Read the model definition and answer for the solid it produces. Units are mm, in the model's axes. A direction names the side the tool comes from. Coordinates: 2 decimals unless noted, no trailing zeros. Write each loop counter-clockwise with the first axis right and the second up, starting at its lowest first coordinate (ties: lowest second). Pieces come first, ordered by that corner, then holes.
Item 1: Section A-A (x = 2.5) is taken. Give the vertices of the cut face in (y, z), then the cut area to 3 significant figures.
Item 2: A tool of negligible diameter and unlimited length cuts with its end or side. For faces 4 (the face through (12, 1, -28)), 5 (the face through (37, 3, -17)), from which of +Z, -Z, +X, -X, +Y, -Y can it reach the whole face along a straight path? Write none if from no direction.
Item 3: This flat-tipped pin is pushed along its axis until it touches: P1, Ø3, axis at x = 71.5, z = -30.5, coming from the -Y side. Where does it stop, or does it pass through?
Item 4: Determine the mould class of faces 1 (the face through (74, 1, -16)), 2 (the face through (36, 0, -17)), 3 (the face through (72.978, 1.014, -30.966)) for opening direction X: released by +X, released by -X, zero draft, split by the parting line, or undercut.
Item 5: Section C-C (x = 61) is taken. Give the vertices of the cut face in (y, z), then the cut area to 3 significant figures.
Item 6: Straight lines are drawn through the part: probe 1 along Z at (x, y) = (71.5, 0.85); probe 2 along X at (y, z) = (1.4, -2.5); probe 3 along X at (y, z) = (0.85, -26). For each, find the intervals that lie inside material, in ascending order.
Item 7: Section B-B (z = -8) is taken. Give the vertices of the cut face in (x, y), then the cut area to 3 significant figures.
from build123d import *

# Parameters (mm, degrees)
SKETCH1_W           = 74
SKETCH1_H           = 33
BOSS_EXTRUDE1_DEPTH = 2
SKETCH2_W           = 62
SKETCH2_H           = 28
BOSS_EXTRUDE2_DEPTH = 1
SKETCH3_R           = 1.55
CUT_EXTRUDE2_DEPTH  = 5
FILLET1_R           = 0.5
FILLET2_R           = 0.5
SKETCH4_W           = 15
SKETCH4_H           = 15
CUT_EXTRUDE3_DEPTH  = 10
FILLET3_R           = 0.5


with BuildPart() as part:
    # Sketch1 → Boss-Extrude1 (new body)
    with BuildSketch(Plane(origin=(0, 0, 0), x_dir=(1, 0, 0), z_dir=(0, 1, 0))):
        with Locations((37, 16.5)):
            Rectangle(SKETCH1_W, SKETCH1_H)
    extrude(amount=BOSS_EXTRUDE1_DEPTH)

    # Sketch2 → Boss-Extrude2 (add)
    with BuildSketch(Plane(origin=(0, 2, 0), x_dir=(1, 0, 0), z_dir=(0, 1, 0))):
        with Locations((37, 16.5)):
            Rectangle(SKETCH2_W, SKETCH2_H)
    extrude(amount=BOSS_EXTRUDE2_DEPTH)

    # Sketch3 → Cut-Extrude2 (cut)
    with BuildSketch(Plane(origin=(0, 2, 0), x_dir=(1, 0, 0), z_dir=(0, 1, 0))):
        with Locations((2.5, 30.5)):
            Circle(SKETCH3_R)
        with Locations((71.5, 2.5)):
            Circle(SKETCH3_R)
        with Locations((2.5, 2.5)):
            Circle(SKETCH3_R)
        with Locations((71.5, 30.5)):
            Circle(SKETCH3_R)
    extrude(amount=-CUT_EXTRUDE2_DEPTH, mode=Mode.SUBTRACT)

    # Fillet1
    fillet1_edges = [part.edges().sort_by_distance(p)[0] for p in [
        (6, 3, -16.5),
        (37, 3, -2.5),
        (68, 3, -16.5),
        (37, 3, -30.5),
    ]]
    fillet(fillet1_edges, radius=FILLET1_R)

    # Fillet2
    fillet2_edges = [part.edges().sort_by_distance(p)[0] for p in [
        (37, 0, -33),
        (74, 0, -16.5),
        (37, 0, 0),
        (0, 0, -16.5),
        (0, 1, -33),
        (74, 1, -33),
        (74, 1, 0),
        (0, 1, 0),
    ]]
    fillet(fillet2_edges, radius=FILLET2_R)

    # Sketch4 → Cut-Extrude3 (cut)
    with BuildSketch(Plane.XZ):
        with Locations((12.5, -20.5)):
            Rectangle(SKETCH4_W, SKETCH4_H)
    extrude(amount=-CUT_EXTRUDE3_DEPTH, mode=Mode.SUBTRACT)

    # Fillet3
    fillet3_edges = [part.edges().sort_by_distance(p)[0] for p in [
        (13.25, 3, -13),
        (20, 1.5, -13),
        (13.25, 3, -28),
        (5, 0, -20.5),
        (12.5, 0, -28),
        (20, 0, -20.5),
        (12.5, 0, -13),
        (6.146446609, 2.853553391, -28),
        (6.146446609, 2.853553391, -13),
        (20, 3, -20.5),
        (5, 2, -20.5),
        (5, 1, -28),
        (6, 2.25, -13),
        (5.5, 2, -13),
        (5, 1, -13),
        (5.5, 2, -28),
        (6, 2.25, -28),
        (20, 1.5, -28),
    ]]
    fillet(fillet3_edges, radius=FILLET3_R)


solid = part.part
Established:
1. outline: (0, -32.5) arc R0.5 ccw to (0.5, -33) - (2, -33) - (2, -32.05) - (0, -32.05) - close; (0, -28.95) - (2, -28.95) - (2, -4.05) - (0, -4.05) - close; (0, -0.95) - (2, -0.95) - (2, 0) - (0.5, 0) arc R0.5 ccw to (0, -0.5) - close
1. area: 53.5 mm2
2. face 4: +Y, -Y
2. face 5: +Z, -Z, +X, -X, +Y
3. P1: passes through
4. face 1: released by +X
4. face 2: zero draft
4. face 3: undercut
5. outline: (0, -32.5) arc R0.5 ccw to (0.5, -33) - (2, -33) - (2, -30.5) - (2.5, -30.5) arc R0.5 ccw to (3, -30) - (3, -3) arc R0.5 ccw to (2.5, -2.5) - (2, -2.5) - (2, 0) - (0.5, 0) arc R0.5 ccw to (0, -0.5) - close
5. area: 93.8 mm2
6. probe 1: z = -33 to -32.05, -28.95 to -4.05, -0.95 to 0
6. probe 2: x = 0 to 0.95, 4.05 to 69.95, 73.05 to 74
6. probe 3: x = 0 to 5, 20 to 74
7. outline: (0, 0.5) arc R0.5 ccw to (0.5, 0) - (73.5, 0) arc R0.5 ccw to (74, 0.5) - (74, 2) - (68, 2) - (68, 2.5) arc R0.5 ccw to (67.5, 3) - (6.5, 3) arc R0.5 ccw to (6, 2.5) - (6, 2) - (0, 2) - close
7. area: 210 mm2
